from build123d import *

# Parameters (mm, degrees)
SKETCH1_W                     = 60
SKETCH1_H                     = 100
BOSS_EXTRUDE1_DEPTH           = 20
SKETCH2_W                     = 32
SKETCH2_H                     = 56
CUT_EXTRUDE1_DEPTH            = 14.325
CUT_EXTRUDE2_DEPTH            = 10
CSK_FOR_M4_SFHCS1_D           = 4.5
CSK_FOR_M4_SFHCS1_CSINK_D     = 8.96
CSK_FOR_M4_SFHCS1_CSINK_ANGLE = 90


with BuildPart() as part:
    # Sketch1 → Boss-Extrude1 (new body)
    with BuildSketch(Plane(origin=(0, 0, 0), x_dir=(1, 0, 0), z_dir=(0, 1, 0))):
        Rectangle(SKETCH1_W, SKETCH1_H)
    extrude(amount=BOSS_EXTRUDE1_DEPTH)

    # Sketch2 → Cut-Extrude1 (cut)
    with BuildSketch(Plane(origin=(0, 20, 0), x_dir=(1, 0, 0), z_dir=(0, 1, 0))):
        with Locations((-14, 22)):
            Rectangle(SKETCH2_W, SKETCH2_H)
    extrude(amount=-CUT_EXTRUDE1_DEPTH, mode=Mode.SUBTRACT)

    # Sketch3 → Cut-Extrude2 (cut)
    with BuildSketch(Plane(origin=(0, 20, 0), x_dir=(1, 0, 0), z_dir=(0, 1, 0))):
        Polygon((30, 50), (12, 50), (12, -16), (-30, -16), (-30, -40), (30, -40), align=None)
    extrude(amount=-CUT_EXTRUDE2_DEPTH, mode=Mode.SUBTRACT)

    # CSK for M4 SFHCS1 (through all)
    with Locations(Plane(origin=(0, 10, 0), x_dir=(1, 0, 0), z_dir=(0, 1, 0))):
        with Locations((20, 40), (10, -30), (-10, -30)):
            CounterSinkHole(CSK_FOR_M4_SFHCS1_D / 2, CSK_FOR_M4_SFHCS1_CSINK_D / 2, counter_sink_angle=CSK_FOR_M4_SFHCS1_CSINK_ANGLE)


solid = part.part
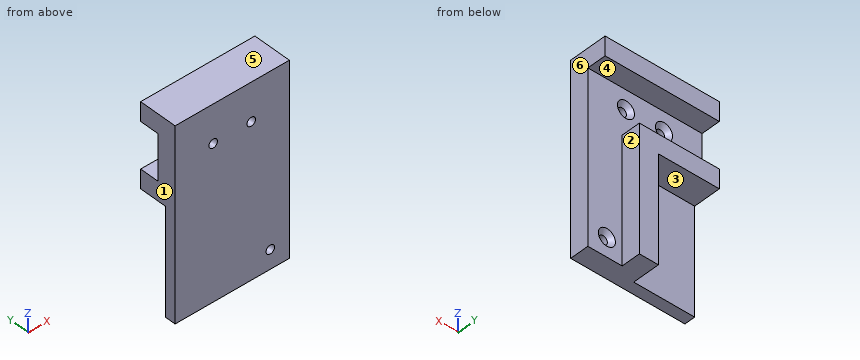
Model file for the job. Use its own axes, mm. Face numbers are marked on the shaded views. A direction names the side the tool comes from. Give positions to 0.01 mm unless a question says otherwise; leave off trailing zeros. Order: outer loops, then holes, each group sorted by start corner. A loop starts at its lowest first (then second) coordinate and runs counter-clockwise, first axis right, second up. Notation, with made-up numbers: M -38,78 L -27,78 A18 ccw -27,112 Z; hole C -21.75,76 d3. An arc over 180 degrees is marked long. Put each result on its own line as item: value. Start each with the question number.
(1) Band-saw the part on A-A on x = -10. Give the cut face in (y, z) (3 decimals).
(2) Band-saw the part on C-C on y = 18.25. Give the cut face in (x, z), then the cut area to 3 significant figures.
(3) Pin check, flat tips, straight feed: pin 1 Ø1 at (x, z) = (21, -15.5) entering from +Y; pin 2 Ø6 at (x, z) = (-15.5, -25) entering from +Y (3 decimals); pin 3 Ø7 at (x, y) = (-19.5, 11) entering from -Z; pin 4 Ø4 at (x, z) = (-10, 30) entering from -Y. Stop position of each tip, or through.
(4) Pull direction Z, two halves, no side cores. Call the marked faces 4, 5 and 6: released by +Z, released by -Z, zero draft, split by the parting line, or undercut.
(5) Band-saw the part on B-B on z = -40. Give the cut face in (x, y) (3 decimals).
(6) Drill centre lines: L1, parallel to X at y = 5.75, z = -40; L2, parallel to X at y = 3.5, z = -40; L3, parallel to Z at x = 10, y = 2.75. Where is each one in solid material? Low to high. Write a range as [from, to].
(7) Tool access for the marked faces 1, 2 and 3: list every direction of +Z, -Z, +X, -X, +Y, -Y with a clear straight run to the whole face (end or side of a thin tool).
(8) Band-saw the part on D-D on z = 30. Give the cut face in (x, y).
Results below:
1. outline: M 0,-50 L 5.675,-50 L 5.675,6 L 20,6 L 20,16 L 10,16 L 10,25.52 L 7.77,27.75 L 0,27.75 Z; M 0,32.25 L 7.77,32.25 L 10,34.48 L 10,40 L 20,40 L 20,50 L 0,50 Z
2. outline: M -30,6 L 2,6 L 2,-50 L 12,-50 L 12,16 L -30,16 Z; M -30,40 L 30,40 L 30,50 L -30,50 Z
2. area: 1,580 mm2
3. pin 1: stops at y = 10
3. pin 2: stops at y = 5.675
3. pin 3: stops at z = 6
3. pin 4: passes through
4. face 4: undercut
4. face 5: released by +Z
4. face 6: zero draft
5. outline: M -30,0 L 17.75,0 L 17.75,7.77 L 15.52,10 L 12,10 L 12,20 L 2,20 L 2,5.675 L -30,5.675 Z; M 22.25,0 L 30,0 L 30,10 L 24.48,10 L 22.25,7.77 Z
6. L1: x = [2, 17.75], [22.25, 30]
6. L2: x = [-30, 17.75], [22.25, 30]
6. L3: z = [-50, 27.75], [32.25, 50]
7. face 1: +Z, -Z, -X, +Y, -Y
7. face 2: -Z, +X, +Y
7. face 3: -Z, -X, +Y
8. outline: M -30,0 L -12.25,0 L -12.25,7.77 L -14.48,10 L -30,10 Z; M -7.75,0 L 7.75,0 L 7.75,7.77 L 5.52,10 L -5.52,10 L -7.75,7.77 Z; M 12.25,0 L 30,0 L 30,10 L 14.48,10 L 12.25,7.77 Z
